For this review, use the dimensioned drawing (mm, ordinates from the lowest corner) and the shaded views. Give positions to 0.01 mm unless a question says otherwise; leave off trailing zeros. Order: outer loops, then holes, each group sorted by start corner. A loop starts at its lowest first (then second) coordinate and runs counter-clockwise, first axis right, second up.
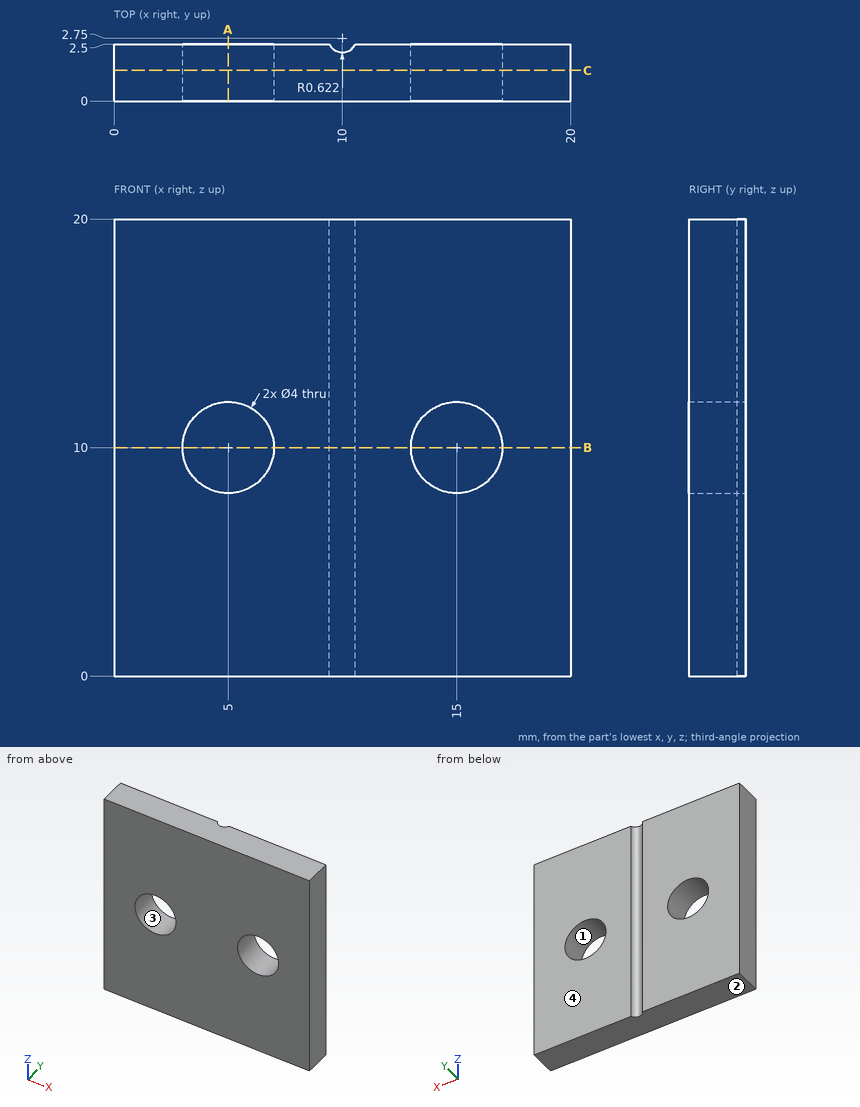
1. Take a section at C-C (y = 1.35). State the section outline as (x, z) points.
Recorded:
outline: (0, 0) - (20, 0) - (20, 20) - (0, 20) - close; hole circle Ø4 at (5, 10); hole circle Ø4 at (15, 10)
2. For line 1 along X through (y, z) = (1, 10); line 2 along Z through (x, y) = (15, 2.05); line 3 along Z through (x, y) = (16.25, 2.25), list the stretches that pass through material, from the lowest coordinate up.
Recorded:
line 1: x = 0 to 3, 7 to 13, 17 to 20
line 2: z = 0 to 8, 12 to 20
line 3: z = 0 to 8.44, 11.56 to 20
3. Draft analysis for pull direction Z (two halves, no side actions). For the marked faces 1, 2, 3 and 4, state which applies: pulls with the +Z half, pulls with the -Z half, needs draft (parallel to the pull), parting line crosses it, or undercut.
Recorded:
face 1: undercut
face 2: pulls with the -Z half
face 3: undercut
face 4: needs draft
4. Take a section at B-B (z = 10). State how many separate pieces and enclosed holes the cut face has, then the cut area to 3 significant figures.
Recorded:
separate pieces: 3
enclosed holes: 0
area: 29.7 mm2
5. For pin 1 (6 mm diameter, centred on x = 17, z = 15, fed in from -Y), flat-tipped, find the tip position at first contact; note if it passes through.
Recorded:
pin 1: stops at y = 0
6. Take a section at A-A (x = 5). State the section outline as (y, z) points.
Recorded:
outline: (0, 0) - (2.5, 0) - (2.5, 8) - (0, 8) - close; (0, 12) - (2.5, 12) - (2.5, 20) - (0, 20) - close
